For this review, take the finished solid that the model builds, in its own axes (mm). A direction names the side the tool comes from. Give positions to 0.01 mm unless a question says otherwise; leave off trailing zeros. Write each loop counter-clockwise with the first axis right and the second up, starting at its lowest first coordinate (ties: lowest second). Pieces come first, ordered by that corner, then holes. Notation, with made-up numbers: (-9, 31.5) -> (4, 31.5) arc R17 ccw to (4, 51.5) -> close; hole circle Ø2 at (-30, -27.5). An arc over 180 degrees is marked (long way). Answer as CSV lines item,"result".
```python
from build123d import *

# Parameters (mm, degrees)
BOSS_EXTRUDE1_DEPTH = 2


with BuildPart() as part:
    # Sketch1 → Revolve1 (revolve)
    with BuildSketch(Plane.XY, mode=Mode.PRIVATE) as revolve1_sk:
        with BuildLine():
            Line((2.5, 14.732142857), (2.5, -18.067857143))
            Line((2.5, -18.067857143), (3.536022963, -18.067857143))
            Line((3.536022963, -18.067857143), (3.536022963, -20.596420744))
            Line((3.536022963, -20.596420744), (1.167881341, -20.596420744))
            Line((1.167881341, -20.596420744), (1.167881341, -18.729405275))
            Line((1.167881341, -18.729405275), (0, -17.565615784))
            Line((0, -17.565615784), (0, 14.932142857))
            Line((0, 14.932142857), (2.384728147, 14.932142857))
            ThreePointArc((2.384728147, 14.932142857), (2.958117238, 14.87838149), (3.515144703, 14.732142857))
            Line((3.515144703, 14.732142857), (2.5, 14.732142857))
        make_face()
    revolve(revolve1_sk.sketch.rotate(Axis((0, 0, 0), (0, 1, 0)), 90), axis=Axis((0, 0, 0), (0, 1, 0)))

    # Sketch2 → Boss-Extrude1 (add)
    with BuildSketch(Plane(origin=(0, 14.932142857, 0), x_dir=(1, 0, 0), z_dir=(0, 1, 0))):
        Polygon((2.460727115, 1.230363557), (0.164837461, 2.746233972), (-2.295889654, 1.515870415), (-2.460727115, -1.230363557), (-0.164837461, -2.746233972), (2.295889654, -1.515870415), align=None)
    extrude(amount=BOSS_EXTRUDE1_DEPTH)

    # Sketch3 → Cut-Revolve1 (revolve, cut)
    with BuildSketch(Plane.XY, mode=Mode.PRIVATE) as cut_revolve1_sk:
        Polygon((1.455321173, 17.272335871), (3.239619089, 16.276214666), (3.239619089, 17.272335871), align=None)
    revolve(cut_revolve1_sk.sketch.rotate(Axis((0, 14.732142857, 0), (0, 1, 0)), 90), axis=Axis((0, 14.732142857, 0), (0, 1, 0)), mode=Mode.SUBTRACT)


solid = part.part
```
Q1. For faces 5 (the flat face through (-1.05, 15.83, -2.14)), 6 (the flat face through (-1.329, 15.831, 1.978)), 7 (the flat face through (1.05, 15.83, 2.14)), list the 3-axis set-ups (+Z, -Z, +X, -X, +Y, -Y) from which the entire face can be reached by the end or side of a thin tool; tool diameter is ignored.
Answer block:
face 5,"-Z, -X, +Y"
face 6,"+Z, -X, +Y"
face 7,"+Z, +X, +Y"
Q2. Clearance check with flat-ended pins moving along their axes: pin 1 (1.5 mm diameter, centred on y = -12.5, z = 1, fed in from -X); pin 2 (2 mm diameter, centred on x = 0, z = 0, fed in from -Y); pin 3 (1 mm diameter, centred on x = -2.5, y = 10.5, fed in from +Z). State where each tip first meets the part, or that it passes through.
Answer block:
pin 1,"stops at x = -2.49"
pin 2,"stops at y = -18.56"
pin 3,"stops at z = 1.5"
Q3. Draft analysis for pull direction X (two halves, no side actions). For faces 1 (the conical face through (0.19, -17.88, 0.25)), 2 (the cylindrical face through (-0.351, -19.65, -1.114)), 3 (the flat face through (1.329, 15.831, -1.978)), 4 (the flat face through (2, 14.732, -2)), state which applies: released by +X, released by -X, zero draft, split by the parting line, or undercut.
Answer block:
face 1,"undercut"
face 2,"undercut"
face 3,"released by +X"
face 4,"zero draft"
Q4. Add section A-A (y = -1). Write out the cut boundary in (x, z), plus the area to 3 significant figures.
Answer block:
outline,"circle Ø5 at (0, 0)"
area,"19.6 mm2"
Q5. To check wall thickness, follow probe 1 along X at (y, z) = (-19.25, 0); probe 2 along Z at (x, y) = (-0.75, -7). State the ranges of each line that lie inside material, in increasing order. Write a range as [from, to].
Answer block:
probe 1,"x = [-3.54, -1.17], [1.17, 3.54]"
probe 2,"z = [-2.38, 2.38]"
